Geometry: see drawing. Coordinates: mm, zero at the bounding-box minimum. Give positions to 0.01 mm unless a question says otherwise; leave off trailing zeros. Write each loop counter-clockwise with the first axis right and the second up, starting at its lowest first coordinate (ties: lowest second). Pieces come first, ordered by that corner, then holes. Notation, with made-up numbers: (4.25, -13) -> (58.25, -13) arc R34 cw to (58.25, 23) -> close; hole circle Ø2 at (63.25, 43). An arc over 180 degrees is marked (long way). Answer as a JSON object with one key per item and string values. Group by question number.
Item 1: Pull-direction query (X, two-part tool) for the marked faces 1, 2 and 3; classes: pulls with the +X half, pulls with the -X half, needs draft (parallel to the pull), parting line crosses it, or undercut.
Item 2: Ray query, probe 1 along Y at (x, z) = (24.5, 10); probe 2 along Z at (x, y) = (21, 10.5). Return the intervals inside material, ascending. Write a range as from..to.
Item 3: Section query A-A on y = 10. Return the cut outline in (x, z), plus the area to 3 significant figures.
Item 4: Section query C-C on x = 13. Return the cut outline in (y, z).
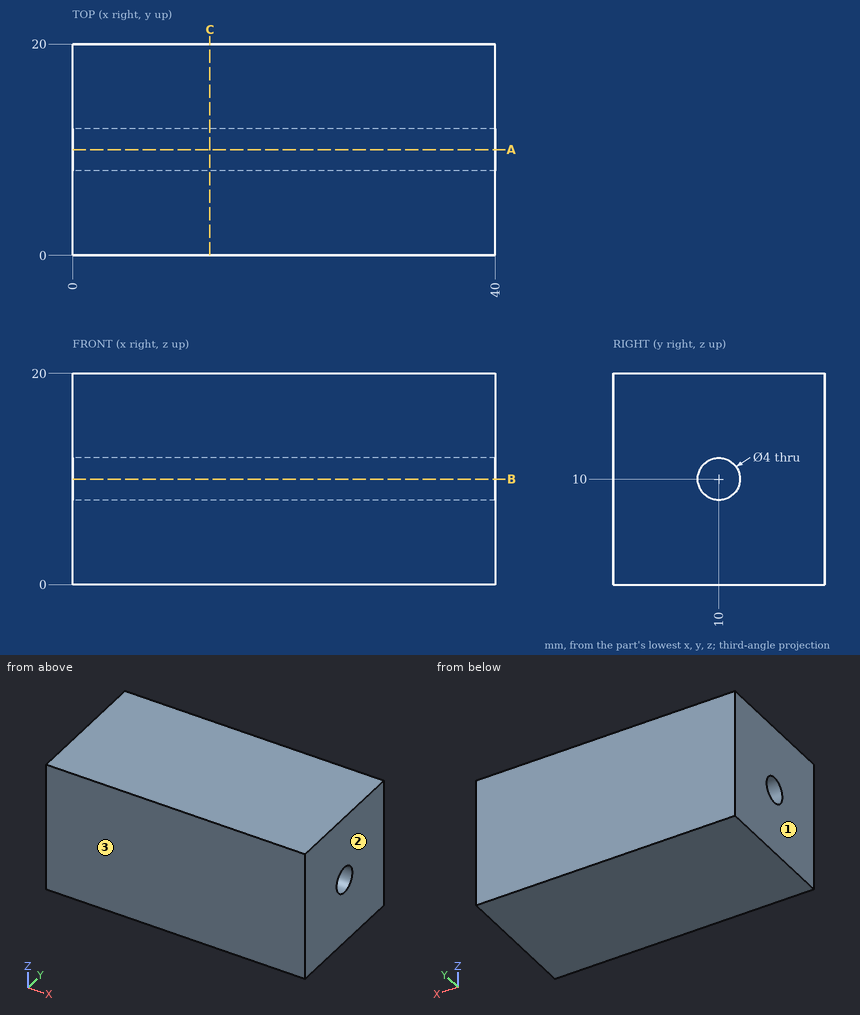
Worked answers:
{
 "1": {"face 1": "pulls with the -X half", "face 2": "pulls with the +X half", "face 3": "needs draft"},
 "2": {"probe 1": "0..8, 12..20", "probe 2": "0..8.06, 11.94..20"},
 "3": {"outline": "(0, 0) -> (40, 0) -> (40, 8) -> (0, 8) -> close; (0, 12) -> (40, 12) -> (40, 20) -> (0, 20) -> close", "area": "640 mm^2"},
 "4": {"outline": "(0, 0) -> (20, 0) -> (20, 20) -> (0, 20) -> close; hole circle Ø4 at (10, 10)"}
}
